Geometry check sheet. Reference: the model listing, model coordinates, mm. A direction names the side the tool comes from. Give positions to 0.01 mm unless a question says otherwise; leave off trailing zeros. Order: outer loops, then holes, each group sorted by start corner. A loop starts at its lowest first (then second) coordinate and runs counter-clockwise, first axis right, second up. Notation, with made-up numbers: M 36,32 L 93,32 A15 ccw 93,41 Z; hole C 5.25,36.5 d6. An arc over 180 degrees is marked long. Put each result on its own line as item: value. Start each with the question number.
Q1. Access from +Z, -Z, +X, -X, +Y, -Y to the whole of each face (thin tool, end or side, straight path). Record for faces 5 (the cylindrical face through (26.76, -0.49, 0.99)), 6 (the flat face through (18, 30, 21)), 7 (the flat face through (17, 44.06, 10)).
Q2. Section check B-B on x = 18. Record the cut outline in (y, z).
Q3. Section check A-A on z = 15.75. Record the cut outline in (x, y).
Q4. Go/stop test with flat-tipped pins: pin 1 (18.5 mm diameter, centred on x = 3.5, y = 21, fed in from +Z); pin 2 (17.5 mm diameter, centred on x = 0, y = -33, fed in from -Z); pin 3 (18 mm diameter, centred on x = 38, y = 0, fed in from -Z). Record where each tip stops, or that it passes through.
Q5. Section check D-D on z = 22.75. Record the cut outline in (x, y).
Q6. Section check C-C on y = -35. Record the cut outline in (x, z).
Q7. Mould release check, pull along Z, two halves, no side actions. Record for faces 1 (the flat face through (15.291, -35, 11)), 2 (the flat face through (15.291, 35, 11)), 3 (the flat face through (4, 29, 18)), 4 (the flat face through (50.291, -1, 10)): +Z half, -Z half, draft (parallel to the pull), parting line (faces both ways), or undercut.
Q8. Material ranges on L1, parallel to Y at x = 0, z = 8.5; L2, parallel to Y at x = 38, z = 18.6; L3, parallel to Y at x = 0, z = 19.95, recorded low to high.
```python
from build123d import *

# Parameters (mm, degrees)
F1_DEPTH  = 2
F2_R      = 9.75
F2_R_2    = 11.25
F2_R_3    = 2
F3_DEPTH  = 16
F4_R      = 9.75
F4_R_2    = 2
F4_R_3    = 5.1
F5_DEPTH  = 3
F7_DEPTH  = 40
F6_R      = 4
F8_DEPTH  = 35
F9_R      = 3.75
F9_R_2    = 1.4
F10_DEPTH = 8


# Not quite as in the source:
# - after a boolean that leaves OpenCascade's solid faulty, fix() repairs it
# - a feature names something its author has since deleted; it is built from what else it names


with BuildPart() as f1:
    # F0 (on Top) → F1 (new body)
    with BuildSketch(Plane.XY):
        with BuildLine():
            Line((50.2909459174, -23.5600714934), (50.2909459174, 23.5599285066))
            Line((50.2909459174, 23.5599285066), (50.2909459174, 39.0599285066))
            ThreePointArc((50.2909459174, 39.0599285066), (48.8264798233, 42.5954624125), (45.2909459174, 44.0599285066))
            Line((45.2909459174, 44.0599285066), (-12, 44.0599285066))
            Line((-12, 44.0599285066), (-12, 0))
            Line((-12, 0), (-12, -44.0599285066))
            Line((-12, -44.0599285066), (45.2909459174, -44.0599285066))
            ThreePointArc((45.2909459174, -44.0599285066), (48.8264798233, -42.5954624125), (50.2909459174, -39.0599285066))
            Line((50.2909459174, -39.0599285066), (50.2909459174, -23.5600714934))
        make_face()
        with BuildLine():
            ThreePointArc((9.75, -33), (-6.8942911166, -39.8942911166), (0, -23.25))
            ThreePointArc((0, -23.25), (6.8942911166, -26.1057088834), (9.75, -33))
        make_face(mode=Mode.SUBTRACT)
        with BuildLine():
            ThreePointArc((9.75, 33), (6.8942911166, 26.1057088834), (0, 23.25))
            ThreePointArc((0, 23.25), (-6.8942911166, 39.8942911166), (9.75, 33))
        make_face(mode=Mode.SUBTRACT)
        with BuildLine():
            ThreePointArc((26.75, 0), (38, 11.25), (49.25, 0))
            ThreePointArc((49.25, 0), (38, -11.25), (26.75, 0))
        make_face(mode=Mode.SUBTRACT)
    extrude(amount=F1_DEPTH)

    # F2 (on face) → F3 (join)
    with BuildSketch(Plane.XY.offset(2)):
        with BuildLine():
            ThreePointArc((50.2909459174, 39.0599285066), (48.8264798233, 42.5954624125), (45.2909459174, 44.0599285066))
            Line((45.2909459174, 44.0599285066), (-12, 44.0599285066))
            Line((-12, 44.0599285066), (-12, -44.0599285066))
            Line((-12, -44.0599285066), (45.2909459174, -44.0599285066))
            ThreePointArc((45.2909459174, -44.0599285066), (48.8264798233, -42.5954624125), (50.2909459174, -39.0599285066))
            Line((50.2909459174, -39.0599285066), (50.2909459174, 39.0599285066))
        make_face()
        with Locations((0, -33)):
            Circle(F2_R, mode=Mode.SUBTRACT)
        with Locations((0, 33)):
            Circle(F2_R, mode=Mode.SUBTRACT)
        with Locations((38, 0)):
            Circle(F2_R_2, mode=Mode.SUBTRACT)
        with Locations((38, 0)):
            Circle(F2_R_2)
        with Locations((38, -8)):
            Circle(F2_R_3, mode=Mode.SUBTRACT)
        with Locations((30, 0)):
            Circle(F2_R_3, mode=Mode.SUBTRACT)
        with BuildLine():
            ThreePointArc((38, 5.1), (41.6062445841, 3.6062445841), (43.1, 0))
            ThreePointArc((43.1, 0), (34.3937554159, -3.6062445841), (38, 5.1))
        make_face(mode=Mode.SUBTRACT)
        with BuildLine():
            ThreePointArc((40, 8), (39.4142135624, 6.5857864376), (38, 6))
            ThreePointArc((38, 6), (36.5857864376, 9.4142135624), (40, 8))
        make_face(mode=Mode.SUBTRACT)
        with BuildLine():
            ThreePointArc((48, 0), (46, -2), (44, 0))
            ThreePointArc((44, 0), (46, 2), (48, 0))
        make_face(mode=Mode.SUBTRACT)
    extrude(amount=F3_DEPTH)

    # F4 (on face) → F5 (join)
    with BuildSketch(Plane.XY.offset(18)):
        with BuildLine():
            Line((50.2909459174, -39.0599285066), (50.2909459174, 39.0599285066))
            ThreePointArc((50.2909459174, 39.0599285066), (48.8264798233, 42.5954624125), (45.2909459174, 44.0599285066))
            Line((45.2909459174, 44.0599285066), (-12, 44.0599285066))
            Line((-12, 44.0599285066), (-12, -44.0599285066))
            Line((-12, -44.0599285066), (45.2909459174, -44.0599285066))
            ThreePointArc((45.2909459174, -44.0599285066), (48.8264798233, -42.5954624125), (50.2909459174, -39.0599285066))
        make_face()
        with Locations((0, -33)):
            Circle(F4_R, mode=Mode.SUBTRACT)
        with Locations((38, -8)):
            Circle(F4_R_2, mode=Mode.SUBTRACT)
        with Locations((0, 33)):
            Circle(F4_R, mode=Mode.SUBTRACT)
        with Locations((30, 0)):
            Circle(F4_R_2, mode=Mode.SUBTRACT)
        with Locations((38, 0)):
            Circle(F4_R_3, mode=Mode.SUBTRACT)
        with Locations((38, 8)):
            Circle(F4_R_2, mode=Mode.SUBTRACT)
        with Locations((46, 0)):
            Circle(F4_R_2, mode=Mode.SUBTRACT)
        with Locations((0, -33)):
            Circle(F4_R)
        with Locations((0, 33)):
            Circle(F4_R)
    extrude(amount=F5_DEPTH)

    # F0 (on Top) → F7 (cut)
    with BuildSketch(Plane.XY):
        with BuildLine():
            ThreePointArc((5.5, -33), (3.8890872965, -29.1109127035), (0, -27.5))
            ThreePointArc((0, -27.5), (-3.8890872965, -36.8890872965), (5.5, -33))
        make_face()
        with BuildLine():
            ThreePointArc((5.5, 33), (-3.8890872965, 36.8890872965), (0, 27.5))
            ThreePointArc((0, 27.5), (3.8890872965, 29.1109127035), (5.5, 33))
        make_face()
    extrude(amount=F7_DEPTH, mode=Mode.SUBTRACT)

    add(f1.part.fix(), mode=Mode.REPLACE)

    # F6 (on face) → F8 (cut)
    with BuildSketch(Plane.YZ.offset(50.2909459174)):
        with Locations((35, 10.5)):
            Circle(F6_R)
        with Locations((-35, 10.5)):
            Circle(F6_R)
    extrude(amount=-F8_DEPTH, mode=Mode.SUBTRACT)

    # F9 (on face) → F10 (join)
    with BuildSketch(Plane.XY.offset(21)):
        with Locations((18, -30.0599285066)):
            Circle(F9_R)
        with Locations((18, -30.0599285066)):
            Circle(F9_R_2, mode=Mode.SUBTRACT)
        with Locations((18, 30.0599285066)):
            Circle(F9_R)
        with Locations((18, 30.0599285066)):
            Circle(F9_R_2, mode=Mode.SUBTRACT)
    extrude(amount=F10_DEPTH)


solid = f1.part
```
Results found:
1. face 5: -Z
1. face 6: +Z
1. face 7: +Z, -Z, +X, -X, +Y
2. outline: M -44.06,0 L 44.06,0 L 44.06,21 L 33.81,21 L 33.81,29 L 31.46,29 L 31.46,21 L 28.66,21 L 28.66,29 L 26.31,29 L 26.31,21 L -26.31,21 L -26.31,29 L -28.66,29 L -28.66,21 L -31.46,21 L -31.46,29 L -33.81,29 L -33.81,21 L -44.06,21 Z; hole C -35,10.5 d8; hole C 35,10.5 d8
3. outline: M -12,-44.06 L 45.29,-44.06 A5 ccw 50.29,-39.06 L 50.29,39.06 A5 ccw 45.29,44.06 L -12,44.06 Z; hole C 0,-33 d19.5; hole C 0,33 d19.5; hole C 30,0 d4; hole C 38,0 d10.2; hole C 38,-8 d4; hole C 38,8 d4; hole C 46,0 d4
4. pin 1: stops at z = 21
4. pin 2: stops at z = 18
4. pin 3: stops at z = 2
5. outline: C 18,-30.06 d7.5; C 18,30.06 d7.5; hole C 18,-30.06 d2.8; hole C 18,30.06 d2.8
6. outline: M -12,0 L -9.54,0 L -9.54,18 L -5.12,18 L -5.12,21 L -12,21 Z; M 5.12,18 L 9.54,18 L 9.54,0 L 50.29,0 L 50.29,6.5 L 15.29,6.5 L 15.29,14.5 L 50.29,14.5 L 50.29,21 L 5.12,21 Z
7. face 1: undercut
7. face 2: undercut
7. face 3: -Z half
7. face 4: draft
8. L1: y = -44.06 to -42.75, -23.25 to 23.25, 42.75 to 44.06
8. L2: y = -44.06 to -10, -6 to -5.1, 5.1 to 6, 10 to 44.06
8. L3: y = -44.06 to -38.5, -27.5 to 27.5, 38.5 to 44.06
